Geometry check sheet. Reference: the model listing, model coordinates, mm. A direction names the side the tool comes from. Coordinates: 2 decimals unless noted, no trailing zeros. Write each loop counter-clockwise with the first axis right and the second up, starting at its lowest first coordinate (ties: lowest second). Pieces come first, ordered by that corner, then holes. Notation, with made-up numbers: (78.5, -12) -> (112.5, -12) arc R28 cw to (112.5, 7) -> close; hole circle Ø2 at (52.25, 56). An arc over 180 degrees is marked (long way). Use a Markdown table: item, result.
```python
from build123d import *

# Parameters (mm, degrees)
ESQUISSE1_R                  = 4.25
ESQUISSE1_R_2                = 1.7
BOSS_EXTRU_1_DEPTH           = 5
ESQUISSE2_R                  = 3
ENL_V_MAT_EXTRU_1_DEPTH      = 3
BOSS_EXTRU_2_DEPTH           = 3
R_P_TITION_CIRCULAIRE1_DEPTH = 3
ESQUISSE4_R                  = 1
BOSS_EXTRU_3_DEPTH           = 2
R_P_TITION_CIRCULAIRE2_COUNT = 6
ENL_V_START                  = -1
ESQUISSE5_R                  = 3
ENL_V_MAT_EXTRU_2_DEPTH      = 1
CONG_1_R                     = 0.2
ESQUISSE6_R                  = 4.5
ESQUISSE6_R_2                = 3.5
ENL_V_MAT_EXTRU_3_DEPTH      = 1
CONG_2_R                     = 0.25


# Read off the part's stored shape, not the designer's step: Répétition circulaire1
with BuildPart() as part:
    # Esquisse1 → Boss.-Extru.1 (new body)
    with BuildSketch(Plane.XY):
        Circle(ESQUISSE1_R)
        Circle(ESQUISSE1_R_2, mode=Mode.SUBTRACT)
    extrude(amount=BOSS_EXTRU_1_DEPTH)

    # Esquisse2 → Enlèv. mat.-Extru.1 (cut)
    with BuildSketch(Plane(origin=(0, 0, 0), x_dir=(-1, 0, 0), z_dir=(0, 0, -1))):
        Circle(ESQUISSE2_R)
    extrude(amount=-ENL_V_MAT_EXTRU_1_DEPTH, mode=Mode.SUBTRACT)

    # Esquisse3 → Boss.-Extru.2 (add)
    with BuildSketch(Plane(origin=(0, 0, 0), x_dir=(-1, 0, 0), z_dir=(0, 0, -1))):
        Polygon((-0.3, 3), (0, 2.6), (0.3, 3), align=None)
    extrude(amount=-BOSS_EXTRU_2_DEPTH)

    # Répétition circulaire1 outline → Répétition circulaire1 (add)
    with BuildSketch(Plane.XY):
        with BuildLine():
            ThreePointArc((1.052468236, 2.80932565), (0.776457135, 2.897777479), (0.493198596, 2.959181499))
            Line((0.493198596, 2.959181499), (0.672929517, 2.511407148))
            Line((0.672929517, 2.511407148), (1.052468236, 2.80932565))
        make_face()
        with BuildLine():
            ThreePointArc((-0.493198596, 2.959181499), (-0.776457135, 2.897777479), (-1.052468236, 2.80932565))
            Line((-1.052468236, 2.80932565), (-0.672929517, 2.511407148))
            Line((-0.672929517, 2.511407148), (-0.493198596, 2.959181499))
        make_face()
        with BuildLine():
            ThreePointArc((-1.242285791, 2.730700645), (-1.5, 2.598076211), (-1.743713233, 2.441201376))
            Line((-1.743713233, 2.441201376), (-1.3, 2.25166605))
            Line((-1.3, 2.25166605), (-1.242285791, 2.730700645))
        make_face()
        with BuildLine():
            ThreePointArc((-1.906713263, 2.316127054), (-2.121320343, 2.121320343), (-2.316127054, 1.906713263))
            Line((-2.316127054, 1.906713263), (-1.838477631, 1.838477631))
            Line((-1.838477631, 1.838477631), (-1.906713263, 2.316127054))
        make_face()
        with BuildLine():
            ThreePointArc((-2.441201376, 1.743713233), (-2.598076211, 1.5), (-2.730700645, 1.242285791))
            Line((-2.730700645, 1.242285791), (-2.25166605, 1.3))
            Line((-2.25166605, 1.3), (-2.441201376, 1.743713233))
        make_face()
        with BuildLine():
            ThreePointArc((-2.809325651, 1.052468236), (-2.897777479, 0.776457135), (-2.959181499, 0.493198596))
            Line((-2.959181499, 0.493198596), (-2.511407148, 0.672929517))
            Line((-2.511407148, 0.672929517), (-2.809325651, 1.052468236))
        make_face()
        with BuildLine():
            ThreePointArc((-2.985999024, 0.289499268), (-3, 0), (-2.985999024, -0.289499268))
            Line((-2.985999024, -0.289499268), (-2.6, 0))
            Line((-2.6, 0), (-2.985999024, 0.289499268))
        make_face()
        with BuildLine():
            ThreePointArc((-2.959181499, -0.493198596), (-2.897777479, -0.776457135), (-2.809325651, -1.052468236))
            Line((-2.809325651, -1.052468236), (-2.511407148, -0.672929517))
            Line((-2.511407148, -0.672929517), (-2.959181499, -0.493198596))
        make_face()
        with BuildLine():
            ThreePointArc((-2.730700645, -1.242285791), (-2.598076211, -1.5), (-2.441201377, -1.743713233))
            Line((-2.441201377, -1.743713233), (-2.25166605, -1.3))
            Line((-2.25166605, -1.3), (-2.730700645, -1.242285791))
        make_face()
        with BuildLine():
            ThreePointArc((-2.316127055, -1.906713263), (-2.121320344, -2.121320344), (-1.906713263, -2.316127055))
            Line((-1.906713263, -2.316127055), (-1.838477631, -1.838477631))
            Line((-1.838477631, -1.838477631), (-2.316127055, -1.906713263))
        make_face()
        with BuildLine():
            ThreePointArc((-1.743713233, -2.441201377), (-1.5, -2.598076211), (-1.242285791, -2.730700645))
            Line((-1.242285791, -2.730700645), (-1.3, -2.25166605))
            Line((-1.3, -2.25166605), (-1.743713233, -2.441201377))
        make_face()
        with BuildLine():
            ThreePointArc((-1.052468236, -2.809325651), (-0.776457135, -2.897777479), (-0.493198596, -2.959181499))
            Line((-0.493198596, -2.959181499), (-0.672929517, -2.511407148))
            Line((-0.672929517, -2.511407148), (-1.052468236, -2.809325651))
        make_face()
        with BuildLine():
            ThreePointArc((-0.289499268, -2.985999024), (0, -3), (0.289499268, -2.985999024))
            Line((0.289499268, -2.985999024), (0, -2.6))
            Line((0, -2.6), (-0.289499268, -2.985999024))
        make_face()
        with BuildLine():
            ThreePointArc((0.493198596, -2.959181499), (0.776457135, -2.897777479), (1.052468236, -2.809325651))
            Line((1.052468236, -2.809325651), (0.672929517, -2.511407148))
            Line((0.672929517, -2.511407148), (0.493198596, -2.959181499))
        make_face()
        with BuildLine():
            ThreePointArc((1.242285791, -2.730700645), (1.5, -2.598076211), (1.743713233, -2.441201377))
            Line((1.743713233, -2.441201377), (1.3, -2.25166605))
            Line((1.3, -2.25166605), (1.242285791, -2.730700645))
        make_face()
        with BuildLine():
            ThreePointArc((1.906713263, -2.316127055), (2.121320344, -2.121320344), (2.316127055, -1.906713263))
            Line((2.316127055, -1.906713263), (1.838477631, -1.838477631))
            Line((1.838477631, -1.838477631), (1.906713263, -2.316127055))
        make_face()
        with BuildLine():
            ThreePointArc((2.441201377, -1.743713233), (2.598076211, -1.5), (2.730700645, -1.242285791))
            Line((2.730700645, -1.242285791), (2.25166605, -1.3))
            Line((2.25166605, -1.3), (2.441201377, -1.743713233))
        make_face()
        with BuildLine():
            ThreePointArc((2.809325651, -1.052468236), (2.897777479, -0.776457135), (2.959181499, -0.493198596))
            Line((2.959181499, -0.493198596), (2.511407148, -0.672929517))
            Line((2.511407148, -0.672929517), (2.809325651, -1.052468236))
        make_face()
        with BuildLine():
            ThreePointArc((2.985999024, -0.289499268), (3, 0), (2.985999024, 0.289499268))
            Line((2.985999024, 0.289499268), (2.6, 0))
            Line((2.6, 0), (2.985999024, -0.289499268))
        make_face()
        with BuildLine():
            ThreePointArc((2.959181499, 0.493198596), (2.897777479, 0.776457135), (2.809325651, 1.052468236))
            Line((2.809325651, 1.052468236), (2.511407148, 0.672929517))
            Line((2.511407148, 0.672929517), (2.959181499, 0.493198596))
        make_face()
        with BuildLine():
            ThreePointArc((2.730700645, 1.242285791), (2.598076211, 1.5), (2.441201376, 1.743713233))
            Line((2.441201376, 1.743713233), (2.25166605, 1.3))
            Line((2.25166605, 1.3), (2.730700645, 1.242285791))
        make_face()
        with BuildLine():
            ThreePointArc((2.316127054, 1.906713263), (2.121320343, 2.121320343), (1.906713263, 2.316127054))
            Line((1.906713263, 2.316127054), (1.838477631, 1.838477631))
            Line((1.838477631, 1.838477631), (2.316127054, 1.906713263))
        make_face()
        with BuildLine():
            ThreePointArc((1.743713233, 2.441201376), (1.5, 2.598076211), (1.242285791, 2.730700645))
            Line((1.242285791, 2.730700645), (1.3, 2.25166605))
            Line((1.3, 2.25166605), (1.743713233, 2.441201376))
        make_face()
    extrude(amount=R_P_TITION_CIRCULAIRE1_DEPTH)

    # Esquisse4 → Boss.-Extru.3 (add)
    with BuildSketch(Plane.XY.offset(5)):
        with BuildLine():
            Line((-1.95061736, 14.441692106), (-3.75, 6.495190528))
            Line((-3.75, 6.495190528), (-3.75, 2))
            Line((-3.75, 2), (0, 3.364888378))
            Line((0, 3.364888378), (3.75, 2))
            Line((3.75, 2), (3.75, 6.495190528))
            Line((3.75, 6.495190528), (1.95061736, 14.441692106))
            ThreePointArc((1.95061736, 14.441692106), (0, 16), (-1.95061736, 14.441692106))
        make_face()
        with Locations((0, 7.5)):
            Circle(ESQUISSE4_R, mode=Mode.SUBTRACT)
        with Locations((0, 10.5)):
            Circle(ESQUISSE4_R, mode=Mode.SUBTRACT)
        with Locations((0, 13.5)):
            Circle(ESQUISSE4_R, mode=Mode.SUBTRACT)
    boss_extru_3 = extrude(amount=-BOSS_EXTRU_3_DEPTH)

    # Répétition circulaire2: Boss.-Extru.3 ×6 about axis
    r_p_tition_circulaire2_axis = Axis((0, 0, 0), (0, 0, 1))
    for i in range(1, R_P_TITION_CIRCULAIRE2_COUNT):
        add(boss_extru_3.rotate(r_p_tition_circulaire2_axis, i * 360 / R_P_TITION_CIRCULAIRE2_COUNT))

    # Esquisse5 → Enlèv. mat.-Extru.2 (cut)
    with BuildSketch(Plane.XY.offset(5).offset(ENL_V_START)):
        Circle(ESQUISSE5_R)
    extrude(amount=ENL_V_MAT_EXTRU_2_DEPTH, mode=Mode.SUBTRACT)

    # Congé1
    cong_1_edges = [part.edges().sort_by_distance(p)[0] for p in [
        (-4.25, 0, 0),
    ]]
    fillet(cong_1_edges, radius=CONG_1_R)

    # Esquisse6 → Enlèv. mat.-Extru.3 (cut)
    with BuildSketch(Plane.XY.offset(5)):
        Circle(ESQUISSE6_R)
        Circle(ESQUISSE6_R_2, mode=Mode.SUBTRACT)
    extrude(amount=-ENL_V_MAT_EXTRU_3_DEPTH, mode=Mode.SUBTRACT)

    # Congé2
    cong_2_edges = [part.edges().sort_by_distance(p)[0] for p in [
        (-3, 0, 5),
        (-4.5, 0, 5),
        (-3.5, 0, 5),
    ]]
    fillet(cong_2_edges, radius=CONG_2_R - 0.0001)  # a hair under: the kernel refuses the full size


solid = part.part
```
Item 1: Tool access check on faces 5 (the flat face through (-10.53, 2.8, 4.01)), 6 (the flat face through (10.45, 2.73, 4.01)), 7 (the cylindrical face through (-9.887, -5.858, 4.014)). Record the directions out of +Z, -Z, +X, -X, +Y, -Y that give a thin tool (end or side, any length) a straight path to the whole face; none if there is none.
Answer block:
| item | result |
|---|---|
| face 5 | +Z, -Z, -X |
| face 6 | +Z, -Z, +X |
| face 7 | +Z, -Z |
Item 2: Depth check by flat-ended pin: P1, Ø1.2, axis at x = 0, y = 10.5, coming from the -Z side; P2, Ø2.5, axis at x = 9.09, y = 5.25, coming from the -Z side. Enter the tip coordinate at first touch or a pass-through.
Answer block:
| item | result |
|---|---|
| P1 | passes through |
| P2 | stops at z = 3 |
Item 3: Mould release check, pull along Y, two halves, no side actions. Record for faces 1 (the cylindrical face through (-13.84, 8.03, 4.01)), 2 (the flat face through (-4, 3, 5)), 3 (the flat face through (-2.84, 10.52, 4.01)), 4 (the cylindrical face through (-0.13, 11.49, 4.01)): +Y half, -Y half, draft (parallel to the pull), parting line (faces both ways), or undercut.
Answer block:
| item | result |
|---|---|
| face 1 | undercut |
| face 2 | draft |
| face 3 | +Y half |
| face 4 | undercut |
Item 4: Thickness scan on L1, parallel to Y at x = -6.25, z = 4.35; L2, parallel to X at y = 3, z = 3.6; L3, parallel to Z at x = -3, y = 7. Record the ranges inside material, lowest first. Write a range as [from, to].
Answer block:
| item | result |
|---|---|
| L1 | y = [-7.27, -4.72], [-2.78, 2.78], [4.72, 7.27] |
| L2 | x = [-10.74, -7.16], [-5.83, 5.83], [7.16, 10.74] |
| L3 | z = [3, 5] |
Item 5: Section check A-A on y = 13.5. Record the boundary of the cut face in (x, z).
Answer block:
| item | result |
|---|---|
| outline | (-2.16, 3) -> (-1, 3) -> (-1, 5) -> (-2.16, 5) -> close; (1, 3) -> (2.16, 3) -> (2.16, 5) -> (1, 5) -> close |
Item 6: Section check B-B on x = -6.5. Record the boundary of the cut face in (y, z).
Answer block:
| item | result |
|---|---|
| outline | (-7.35, 3) -> (-4.75, 3) -> (-4.75, 5) -> (-7.35, 5) -> close; (-2.75, 3) -> (2.75, 3) -> (2.75, 5) -> (-2.75, 5) -> close; (4.75, 3) -> (7.35, 3) -> (7.35, 5) -> (4.75, 5) -> close |
